Autodesk Inventor part; units mm, degrees
ref_plane "YZ Plane" through (0, 0, 0) normal (1, 0, 0) x (0, 1, 0)
ref_plane "XZ Plane" through (0, 0, 0) normal (0, 1, 0) x (-1, 0, 0)
ref_plane "XY Plane" through (0, 0, 0) normal (0, 0, 1) x (1, 0, 0)
sketch "BodySketch" plane through (0, 0, 0) normal (0, 1, 0) x (-1, 0, 0)
  circle A0 centre (0, 0) radius 18
  dimension "EncoderWheelInterface_Diameter" = 36
extrude "Body" add sketch "BodySketch" along normal blind 9
sketch "FasteningHoleSketch" plane through (0, 9, 0) normal (0, 1, 0) x (1, 0, 0)
  circle A0 centre (0, 0) radius 18
  circle A1 centre (0, 9.5) radius 1.5
  line L0 (0, 0) -> (0, 20.8166) construction
  circle A2 centre (-6.7175, 6.7175) radius 1.5
  circle A3 centre (-9.5, 0) radius 1.5
  circle A4 centre (-6.7175, -6.7175) radius 1.5
  circle A5 centre (0, -9.5) radius 1.5
  circle A6 centre (6.7175, -6.7175) radius 1.5
  circle A7 centre (9.5, 0) radius 1.5
  circle A8 centre (6.7175, 6.7175) radius 1.5
  dimension "d3" = 9.5
  dimension "EncoderWheelInterface_FasteningHole_Diameter" = 3
  dimension "d7" = 360
sketch "ShaftHoleSketch" plane through (0, 9, 0) normal (0, 1, 0) x (1, 0, 0)
  circle A0 centre (0, 0) radius 18
  arc A1 (2.3238, -2.2) -> (-2.3238, -2.2) centre (0, 0) ccw
  line L0 (-2.3238, -2.2) -> (2.3238, -2.2)
  dimension "d11" = 6.4
  dimension "d12" = 1
extrude "ShaftHole" cut sketch "ShaftHoleSketch" against normal up to next contours L0 A1
extrude "FasteningHole" cut sketch "FasteningHoleSketch" against normal up to next contours A1 | A2 | A3 | A4 | A6 | A7 | A8
sketch "MeplatSketch" plane through (0, 9, 0) normal (0, 1, 0) x (1, 0, 0)
  line L0 (2.3238, -2.2) -> (-2.3238, -2.2)
  circle A0 centre (0, 0) radius 18
  line L1 (-7.846, -16.2) -> (7.846, -16.2)
  dimension "d19" = 14
extrude "Metplat" cut sketch "MeplatSketch" against normal up to next contours L1 A0 picked at (-1.3416, -16.6481)
sketch "MeplatHoleSketch" plane through (-7.846, 9, 16.2) normal (0, 0, 1) x (1, 0, 0)
  line L0 (0, -9) -> (15.692, 0) construction
  line L1 (0, 0) -> (15.692, -9) construction
  circle A0 centre (7.846, -4.5) radius 1.5
  point P0 (7.846, -9)
  dimension "EncoderWheelInterface_MeplatHole_Diameter" = 3
extrude "MeplatHole" cut sketch "MeplatHoleSketch" against normal up to surface (14 mm away)
thread "Thread1"
hole "Hole1" at (1.7243, 9, 8.8194) direction (0, -1, 0) diameter 2.459 end through all
equation "\"d3\" = EncoderWheel_FasteningHole_DistanceToCenter"
equation "\"d11\" = Encoder_Shaft_Diameter + EncoderWheelInterface_Margin"
equation "\"d12\" = Encoder_Shaft_Meplat_Depth"
equation "\"EncoderWheelInterface_Margin\" = 0.4"
properties part number "EncoderWheelInterface" material "Polyethylene, High Density"
Geometry: final body of the model. Coordinates: model frame, mm. A direction names the side the tool comes from. Round coordinates to 2 decimals unless told otherwise and drop trailing zeros. Loops run counter-clockwise (first coordinate to the right, second up) from the corner with the lowest first, then second, coordinate; pieces in that order, holes last. Notation, with made-up numbers: M 55.25,-39.5 L 112.25,-39.5 A18 cw 112.25,-31.5 Z; hole C 82.25,15.5 d6. An arc over 180 degrees is marked long. Put each result on its own line as item: value. Start each with the question number.
(1) Material intervals for line 1 along X through (y, z) = (6.5, 0); line 2 along Z through (x, y) = (6, 5.75); line 3 along X through (y, z) = (8, 5.5), sorted ascending. Write a range as [from, to].
(2) Section query A-A (x = 0). Return loops of the section in (y, z), then the cut area to 3 significant figures.
(3) Section query B-B (z = -10). Return loops of the section in (x, y), then the cut area to 3 significant figures.
(4) Section query D-D (x = -9.5). Return loops of the section in (y, z), then the cut area to 3 significant figures.
(5) Draft query along X for faces 3 (the face through (-0.678, 4.437, -17.987)), 4 (the face through (0, 9, 3)), 5 (the face through (-1, 6, 2.2)). Return one class per face: +X half, -X half, draft (parallel to the pull), parting line (faces both ways), or undercut.
(6) Set-up query: faces 1 (the face through (-5.287, 4.563, 6.267)), 2 (the face through (-1.5, 4.57, 9.3)). Return all of +Z, -Z, +X, -X, +Y, -Y with unobstructed straight access to the full face (end or side cutting, diameter ignored); none if empty.
(7) Contact query for flat-ended pins moving along their axis: pin 1 Ø5 at (y, z) = (2.5, -13) entering from +X; pin 2 Ø3 at (y, z) = (5, -3) entering from -X; pin 3 Ø1.4 at (x, y) = (-1, 4.5) entering from -Z. Output: stop coordinate, or through.
(8) Section query C-C (y = 3.5). Return loops of the section in (x, z).
Findings below:
1. line 1: x = [-18, -11], [-8, -3.2], [3.2, 8], [11, 18]
1. line 2: z = [-16.97, -8.03], [-5.4, 5.4], [8.03, 16.2]
1. line 3: x = [-17.14, -7.59], [-5.84, 5.84], [7.59, 17.14]
2. outline: M 0,-18 L 9,-18 L 9,-11 L 0,-11 Z; M 0,-8 L 9,-8 L 9,-3.2 L 0,-3.2 Z; M 0,2.2 L 3,2.2 L 3,16.2 L 0,16.2 Z; M 6,2.2 L 9,2.2 L 9,16.2 L 6,16.2 Z
2. area: 190 mm2
3. outline: M -14.97,0 L -1.41,0 L -1.41,9 L -14.97,9 Z; M 1.41,0 L 14.97,0 L 14.97,9 L 1.41,9 Z
3. area: 244 mm2
4. outline: M 0,-15.29 L 9,-15.29 L 9,-1.5 L 0,-1.5 Z; M 0,1.5 L 9,1.5 L 9,15.29 L 0,15.29 Z
4. area: 248 mm2
5. face 3: parting line
5. face 4: draft
5. face 5: undercut
6. face 1: +Y, -Y
6. face 2: +Z
7. pin 1: stops at x = 14.62
7. pin 2: stops at x = -17.94
7. pin 3: stops at z = -18
8. outline: M -7.85,16.2 A18 ccw long 7.85,16.2 L 1.12,16.2 L 1.12,9.89 A1.23 cw long 1.12,7.75 L 1.12,2.2 L 2.32,2.2 A3.2 cw long -2.32,2.2 L -1.12,2.2 L -1.12,16.2 Z; hole C -9.5,0 d3; hole C -6.72,-6.72 d3; hole C -6.72,6.72 d3; hole C 0,-9.5 d3; hole C 6.72,-6.72 d3; hole C 6.72,6.72 d3; hole C 9.5,0 d3
